Geometry: see drawing. Coordinates: mm, zero at the bounding-box minimum. Give positions to 0.01 mm unless a question says otherwise; leave off trailing zeros. Write each loop counter-clockwise with the first axis right and the second up, starting at its lowest first coordinate (ties: lowest second). Pieces come first, ordered by that corner, then holes. Notation, with made-up numbers: M 49.5,2 L 89.5,2 A15 ccw 89.5,18 Z; hole C 28.5,86.25 d6. An arc over 180 degrees is marked long. Use a Markdown table: item, result. Add a question column.
1) Section C-C on x = 8. Return the cut outline in (y, z).
2) Section A-A on x = 45. Return the cut outline in (y, z), then the cut area to 3 significant figures.
3) Section B-B on y = 1.05. Return the cut outline in (x, z).
4) Section D-D on z = 26.5. Return the cut outline in (x, y), then the cut area to 3 significant figures.
5) Line query: line 1 (Z direction, x = 8, y = 1.1); line 2 (Z direction, x = 9, y = 2.2); line 3 (X direction, y = 2, z = 20). Output: solid intervals per line, ascending.
6) Pin query (flat end, axial travel): pin 1 (1.5 mm diameter, centred on x = 37, z = 34.5, fed in from -Y). Return the tip coordinate at first contact, or that it passes through.
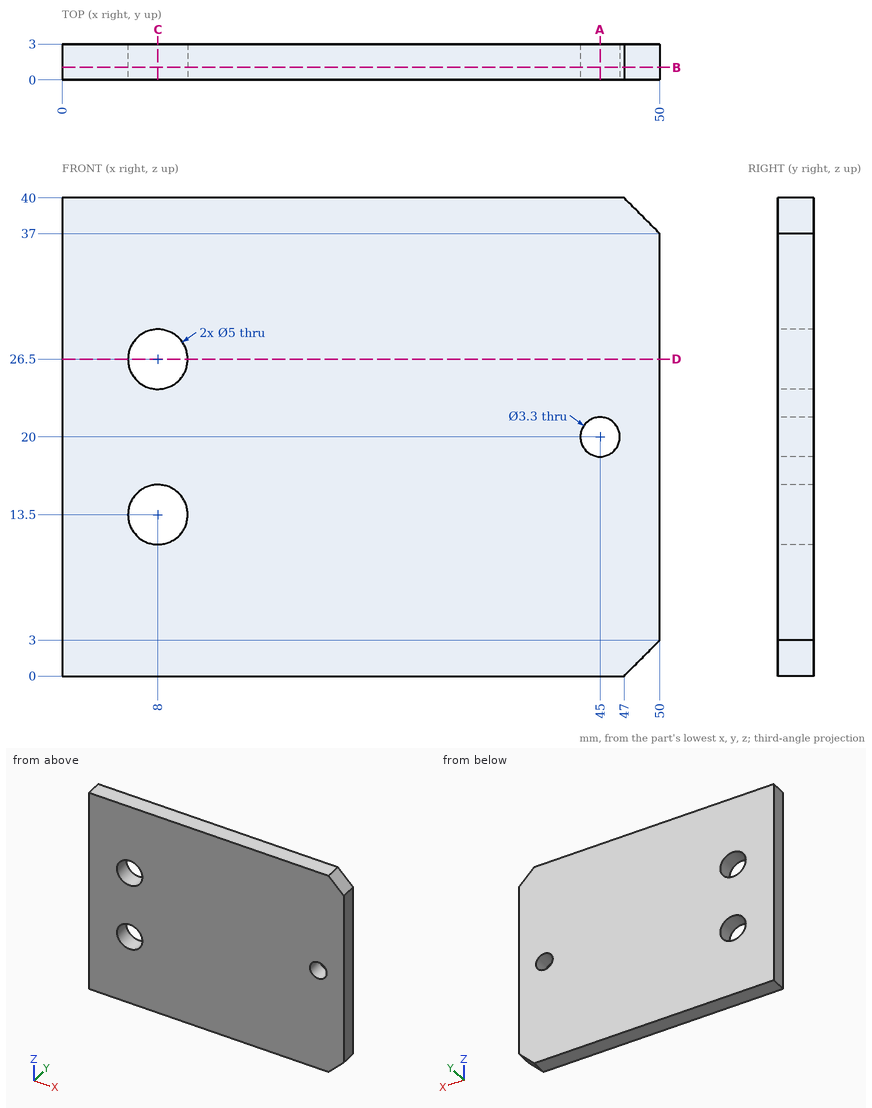
Found:
| question | item | result |
|---|---|---|
| 1 | outline | M 0,0 L 3,0 L 3,11 L 0,11 Z; M 0,16 L 3,16 L 3,24 L 0,24 Z; M 0,29 L 3,29 L 3,40 L 0,40 Z |
| 2 | outline | M 0,0 L 3,0 L 3,18.35 L 0,18.35 Z; M 0,21.65 L 3,21.65 L 3,40 L 0,40 Z |
| 2 | area | 110 mm² |
| 3 | outline | M 0,0 L 47,0 L 50,3 L 50,37 L 47,40 L 0,40 Z; hole C 8,13.5 d5; hole C 8,26.5 d5; hole C 45,20 d3.3 |
| 4 | outline | M 0,0 L 5.5,0 L 5.5,3 L 0,3 Z; M 10.5,0 L 50,0 L 50,3 L 10.5,3 Z |
| 4 | area | 135 mm² |
| 5 | line 1 | 0 to 11, 16 to 24, 29 to 40 |
| 5 | line 2 | 0 to 11.21, 15.79 to 24.21, 28.79 to 40 |
| 5 | line 3 | 0 to 43.35, 46.65 to 50 |
| 6 | pin 1 | y = 0 |
